Verification items for the finished model (mm, model axes). A direction names the side the tool comes from. Give positions to 0.01 mm unless a question says otherwise; leave off trailing zeros. Order: outer loops, then holes, each group sorted by start corner. A loop starts at its lowest first (then second) coordinate and runs counter-clockwise, first axis right, second up. Notation, with made-up numbers: (-31.75, 53.5) -> (3.25, 53.5) arc R33 cw to (3.25, 84.5) -> close; hole circle Ø4 at (43, 20). An arc over 180 degrees is marked (long way). Return JSON: item names as keys, results as strings. Group by question number.
(1) Release check for a two-part mould opening along Z. For faces 1 (the face through (30, 15, 15)), 2 (the face through (25.672, 3.222, 13.946)), 3 (the face through (18, 12, 30)) record: pulls with the +Z half, pulls with the -Z half, needs draft (parallel to the pull), parting line crosses it, or undercut.
(2) Cross-section at D-D on z = 15.5. State how many separate pieces and enclosed holes the cut face has, then the cut area to 3 significant figures.
(3) Thickness scan on line 1 along Z through (x, y) = (5, 26.5); line 2 along Y through (x, z) = (12, 11.5). Record the ranges inside material, lowest first.
(4) Depth check by flat-ended pin: pin 1 Ø2 at (x, z) = (25, 5) entering from +Y; pin 2 Ø3 at (x, z) = (5, 25) entering from +Y. Enter the tip coordinate at first touch or a pass-through.
(5) Cross-section at B-B on x = 12. Enter the section's corners in (y, z).
(6) Cross-section at C-C on z = 9. Enter the section's corners in (x, y), then the cut area to 3 significant figures.
(7) Tool access check on faces 4 (the face through (15, 0, 15)), 5 (the face through (6.22, 25.73, 5.27)). Record the directions out of +Z, -Z, +X, -X, +Y, -Y that give a thin tool (end or side, any length) a straight path to the whole face; none if there is none.
(8) Cross-section at A-A on y = 16.8. Enter the section's corners in (x, z).
from build123d import *

# Parameters (mm, degrees)
SCHIZZO1_W                      = 30
SCHIZZO1_H                      = 30
SCHIZZO1_R                      = 7.5
ESTRUSIONE_ESTRUSIONE1_DEPTH    = 30
FORO_8_0_8_1_D                  = 8
FORO_8_0_8_1_DEPTH              = 10
FORO_8_0_8_1_TIP                = 2.403442476
FORO_FILETTATO_M3_1_AT_2_COUNT  = 2
FORO_FILETTATO_M3_1_AT_2_PITCH  = 20
FORO_FILETTATO_M3_2_D           = 2.5
FORO_FILETTATO_M3_2_DEPTH       = 8.5
FORO_FILETTATO_M3_2_CSINK_D     = 3.05
FORO_FILETTATO_M3_2_CSINK_ANGLE = 120
FORO_FILETTATO_M3_2_TIP         = 0.751075774


with BuildPart() as part:
    # Schizzo1 → Estrusione-Estrusione1 (new body)
    with BuildSketch(Plane.XY):
        with Locations((15, 15)):
            Rectangle(SCHIZZO1_W, SCHIZZO1_H)
        with Locations((12, 16.8)):
            Circle(SCHIZZO1_R, mode=Mode.SUBTRACT)
    extrude(amount=ESTRUSIONE_ESTRUSIONE1_DEPTH)

    # Foro Ø8.0 (8)-1
    with Locations(Plane(origin=(30, 0, 0), x_dir=(0, 0, -1), z_dir=(1, 0, 0))):
        with Locations((-15, 10)):
            Hole(FORO_8_0_8_1_D / 2, depth=FORO_8_0_8_1_DEPTH)
            with Locations((0, 0, -(FORO_8_0_8_1_DEPTH + FORO_8_0_8_1_TIP / 2))):  # 118° drill point
                Cone(0, FORO_8_0_8_1_D / 2, FORO_8_0_8_1_TIP, mode=Mode.SUBTRACT)

    # Schizzo7 → Foro filettato M3-1 (revolve, cut)
    with BuildSketch(Plane(origin=(5, 30, 25), x_dir=(0, 0, 1), z_dir=(1, 0, 0))):
        Polygon((0, 0), (0, 9.251075774), (1.25, 8.5), (1.25, 0.158771324), (1.525, 0), align=None)
    foro_filettato_m3_1 = revolve(axis=Axis((5, 36.35, 25), (0, -1, 0)), mode=Mode.SUBTRACT)

    # Foro filettato M3-1 at 2: Foro filettato M3-1 ×2
    with Locations(*[(i * FORO_FILETTATO_M3_1_AT_2_PITCH, 0, 0) for i in range(1, FORO_FILETTATO_M3_1_AT_2_COUNT)]):
        add(foro_filettato_m3_1, mode=Mode.SUBTRACT)

    # Specchia1: Foro filettato M3-1 across plane
    add(foro_filettato_m3_1.mirror(Plane.XY.offset(15)), mode=Mode.SUBTRACT)

    # Specchia1 copy 1 sketch → Specchia1 copy 1 (revolve, cut)
    with BuildSketch(Plane(origin=(25, 30, 5), x_dir=(0, 0, -1), z_dir=(1, 0, 0))):
        Polygon((0, 0), (0, -9.251075774), (1.25, -8.5), (1.25, -0.158771324), (1.525, 0), align=None)
    revolve(axis=Axis((25, 36.35, 5), (0, 1, 0)), mode=Mode.SUBTRACT)

    # Foro filettato M3-2
    with Locations(Plane(origin=(0, 0, 0), x_dir=(-1, 0, 0), z_dir=(0, -1, 0))):
        with Locations((-25, -15)):
            CounterSinkHole(FORO_FILETTATO_M3_2_D / 2, FORO_FILETTATO_M3_2_CSINK_D / 2, depth=FORO_FILETTATO_M3_2_DEPTH, counter_sink_angle=FORO_FILETTATO_M3_2_CSINK_ANGLE)
            with Locations((0, 0, -(FORO_FILETTATO_M3_2_DEPTH + FORO_FILETTATO_M3_2_TIP / 2))):  # 118° drill point
                Cone(0, FORO_FILETTATO_M3_2_D / 2, FORO_FILETTATO_M3_2_TIP, mode=Mode.SUBTRACT)


solid = part.part
Verdict:
{
 "1": {"face 1": "needs draft", "face 2": "undercut", "face 3": "pulls with the +Z half"},
 "2": {"separate pieces": "2", "enclosed holes": "1", "area": "621 mm²"},
 "3": {"line 1": "0 to 3.75, 6.25 to 23.75, 26.25 to 30", "line 2": "0 to 9.3, 24.3 to 30"},
 "4": {"pin 1": "y = 21.35", "pin 2": "y = 29.99"},
 "5": {"outline": "(0, 0) -> (9.3, 0) -> (9.3, 30) -> (0, 30) -> close; (24.3, 0) -> (30, 0) -> (30, 30) -> (24.3, 30) -> close"},
 "6": {"outline": "(0, 0) -> (30, 0) -> (30, 30) -> (0, 30) -> close; hole circle Ø15 at (12, 16.8)", "area": "723 mm²"},
 "7": {"face 4": "+Z, -Z, +X, -X, -Y", "face 5": "+Y"},
 "8": {"outline": "(0, 0) -> (4.5, 0) -> (4.5, 30) -> (0, 30) -> close; (19.5, 0) -> (30, 0) -> (30, 30) -> (19.5, 30) -> close"}
}
